from build123d import *

# Parameters (mm, degrees)
SKETCH8_R   = 0.45
SKETCH8_R_2 = 0.3


with BuildPart() as part:
    # Sweep1: sweep along a path in Sketch7
    with BuildLine(Plane.XY) as sweep1_path:
        Line((0, 0), (0, 24.171572875))
        ThreePointArc((0, 24.171572875), (0.152240935, 24.93693974), (0.585786438, 25.585786438))
        Line((0.585786438, 25.585786438), (5.656854249, 30.656854249))
    # Sketch8 → Sweep1 (sweep)
    with BuildSketch(Plane(origin=(0, 0, 0), x_dir=(1, 0, 0), z_dir=(0, 1, 0))):
        Circle(SKETCH8_R)
        Circle(SKETCH8_R_2, mode=Mode.SUBTRACT)
    sweep(path=sweep1_path.line)

    # Sketch9 → Cut-Revolve3 (revolve, cut)
    with BuildSketch(Plane.XY, mode=Mode.PRIVATE) as cut_revolve3_sk:
        Polygon((5.579208536, 29.942812433), (5.975052301, 30.338656198), (5.868986284, 30.444722215), align=None)
    revolve(cut_revolve3_sk.sketch.rotate(Axis((6.207317526, 31.207317526, 0), (-0.7071067811865472, -0.7071067811865479, 0)), 180), axis=Axis((6.207317526, 31.207317526, 0), (-0.7071067811865472, -0.7071067811865479, 0)), mode=Mode.SUBTRACT)


solid = part.part
Model file for the job. Use its own axes, mm. Coordinates: 2 decimals unless noted, no trailing zeros. Write each loop counter-clockwise with the first axis right and the second up, starting at its lowest first coordinate (ties: lowest second). Pieces come first, ordered by that corner, then holes. Notation, with made-up numbers: (37, 79) -> (45, 79) arc R15 cw to (45, 92) -> close; hole circle Ø5 at (39, -7.75). An arc over 180 degrees is marked (long way). One line per item, written item: value. Start each with the question number.
1) Pull direction X, two halves, no side cores. Call faces 1 (the face through (3.4, 28, -0.1)), 2 (the face through (0.21, 12.25, 0.4)): +X half, -X half, draft (parallel to the pull), parting line (faces both ways), or undercut.
2) Slice it at B-B on y = 22.5. Write the cut outline in (x, z).
3) Probe probe 1 along X at (y, z) = (18, 0); probe 2 along Y at (x, z) = (2.75, 0.1); probe 3 along Y at (x, z) = (2, 0). List the from-to ranges inside material, lowest first.
4) Slice it at A-A on z = 0. Write the cut outline in (x, y), then the cut area to 3 significant figures.
Answers follow:
1. face 1: undercut
1. face 2: parting line
2. outline: circle Ø0.9 at (0, 0); hole circle Ø0.6 at (0, 0)
3. probe 1: -0.45 to -0.3, 0.3 to 0.45
3. probe 2: 27.13 to 27.35, 28.15 to 28.37
3. probe 3: 26.36 to 26.58, 27.42 to 27.64
4. outline: (-0.45, 0) -> (-0.3, 0) -> (-0.3, 24.17) arc R2.3 cw to (0.37, 25.8) -> (5.44, 30.87) -> (4.94, 30.58) -> (0.27, 25.9) arc R2.45 ccw to (-0.45, 24.17) -> close; (0.3, 0) -> (0.45, 0) -> (0.45, 24.17) arc R1.55 cw to (0.9, 25.27) -> (5.58, 29.94) -> (5.87, 30.44) -> (0.8, 25.37) arc R1.7 ccw to (0.3, 24.17) -> close
4. area: 9.79 mm2
